from build123d import *

# Parameters (mm, degrees)
F1_DEPTH = 57.15
F2_R     = 3.175
F3_R     = 28.57499
F4_R     = 28.575
F5_R     = 28.57499
F7_D     = 15.875
F8_D     = 25.4
F8_DEPTH = 38.1
F8_TIP   = 7.6309298617
F9_D     = 25.4


# Not quite as in the source:
# - a fillet or chamfer is up to 0.001 mm smaller than in the source, because OpenCascade refuses the exact size
# - a length typed as a fraction of an inch, garbled in the dataset ("3 / 203.2 mm" for 3/8 in), is restored


with BuildPart() as f1:
    # F0 (on Top) → F1 (new body)
    with BuildSketch(Plane.XY):
        with BuildLine():
            ThreePointArc((28.575, -6.35), (30.4348719395, -1.8598719395), (34.925, 0))
            Line((34.925, 0), (609.6, 0))
            Line((609.6, 0), (609.6, 15.875))
            Line((609.6, 15.875), (34.925, 15.875))
            ThreePointArc((34.925, 15.875), (30.4348719395, 17.7348719395), (28.575, 22.225))
            Line((28.575, 22.225), (28.575, 36.5125))
            Line((28.575, 36.5125), (0, 36.5125))
            Line((0, 36.5125), (-28.575, 36.5125))
            Line((-28.575, 36.5125), (-28.575, 22.225))
            ThreePointArc((-28.575, 22.225), (-30.4348719395, 17.7348719395), (-34.925, 15.875))
            Line((-34.925, 15.875), (-304.8, 15.875))
            Line((-304.8, 15.875), (-304.8, 0))
            Line((-304.8, 0), (-34.925, 0))
            ThreePointArc((-34.925, 0), (-30.4348719395, -1.8598719395), (-28.575, -6.35))
            Line((-28.575, -6.35), (-28.575, -20.6375))
            Line((-28.575, -20.6375), (0, -20.6375))
            Line((0, -20.6375), (28.575, -20.6375))
            Line((28.575, -20.6375), (28.575, -6.35))
        make_face()
    extrude(amount=F1_DEPTH)

    # F2
    f2_edges = [f1.edges().sort_by_distance(p)[0] for p in [
        (28.575, 36.5125, 28.575),
        (0, 36.5125, 57.15),
        (-28.575, 36.5125, 28.575),
        (0, 36.5125, 0),
        (-28.575, -20.6375, 28.575),
        (0, -20.6375, 57.15),
        (28.575, -20.6375, 28.575),
        (0, -20.6375, 0),
    ]]
    fillet(f2_edges, radius=F2_R)

    # F3 (radius 28.575 in the source; OpenCascade refuses exactly that, so slightly less here)
    f3_edges = [f1.edges().sort_by_distance(p)[0] for p in [
        (-304.8, 7.9375, 57.15),
        (-304.8, 7.9375, 0),
    ]]
    fillet(f3_edges, radius=F3_R)

    # F4
    f4_edges = [f1.edges().sort_by_distance(p)[0] for p in [
        (609.6, 7.9375, 57.15),
    ]]
    fillet(f4_edges, radius=F4_R)

    # F5 (radius 28.575 in the source; OpenCascade refuses exactly that, so slightly less here)
    f5_edges = [f1.edges().sort_by_distance(p)[0] for p in [
        (609.6, 7.9375, 0),
    ]]
    fillet(f5_edges, radius=F5_R)

    # F7 (through all)
    with Locations(Plane.XZ):
        with Locations((-215.9, 28.575)):
            Hole(F7_D / 2)

    # F8 (one way)
    with BuildSketch(Plane.XZ):
        with Locations((0, 28.575)):
            Circle(F8_D / 2)
    extrude(amount=-F8_DEPTH, mode=Mode.SUBTRACT)
    with Locations(Plane.XZ):
        with Locations((0, 28.575)):
            with Locations((0, 0, -(F8_DEPTH + F8_TIP / 2))):  # 118° drill point
                Cone(0, F8_D / 2, F8_TIP, mode=Mode.SUBTRACT)

    # F9 (through all)
    with Locations(Plane(origin=(0, 0, 0), x_dir=(1, 0, 0), z_dir=(0, 1, 0))):
        with Locations((0, -28.575)):
            Hole(F9_D / 2)


solid = f1.part
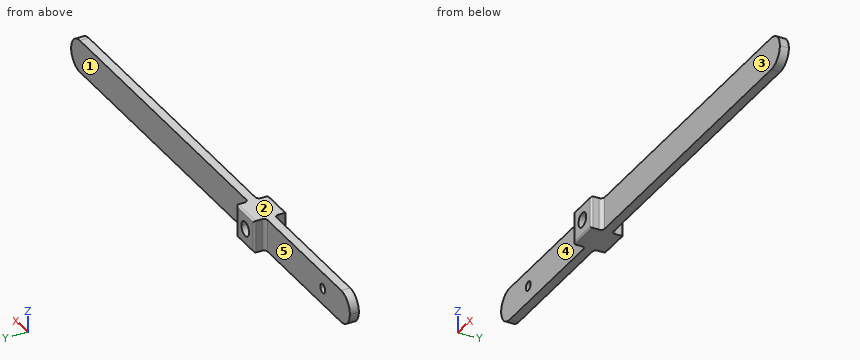
Source: CAD feature listing. Evaluate the final solid. Frame: model axes, mm. Face numbers are marked on the shaded views. A direction names the side the tool comes from. Round coordinates to 2 decimals unless told otherwise and drop trailing zeros. One line per item, written item: value. Start each with the question number.
Item 1: Ray query, L1, parallel to X at y = 7, z = 33.5; L2, parallel to Z at x = 0, y = -6 (3 decimals); L3, parallel to Z at x = -215.9, y = 9. Return the intervals inside material, ascending. Write a range as from..to.
Item 2: Pin query (flat end, axial travel): pin 1 (2 mm diameter, centred on x = 487.5, z = 29.5, fed in from -Y); pin 2 (6 mm diameter, centred on y = -9.5, z = 41, fed in from -X) (3 decimals); pin 3 (9.5 mm diameter, centred on x = -215.9, z = 28.575, fed in from -Y); pin 4 (5.5 mm diameter, centred on y = -9, z = 15.5, fed in from +X). Return the tip coordinate at first contact, or that it passes through.
Item 3: Set-up query: the marked faces 1, 2, 3, 4 and 5. Return all of +Z, -Z, +X, -X, +Y, -Y with unobstructed straight access to the full face (end or side cutting, diameter ignored); none if empty.
Result set:
1. L1: x = -304.37..-222.12, -209.68..-11.71, 11.71..609.17
1. L2: z = 0..15.875, 41.275..57.15
1. L3: z = 0..20.64, 36.51..57.15
2. pin 1: stops at y = 0
2. pin 2: stops at x = -28.575
2. pin 3: passes through
2. pin 4: stops at x = 28.58
3. face 1: +Z, -Z, +X, +Y
3. face 2: +Z, +X, -X, +Y, -Y
3. face 3: +Z, -Z, +X, -Y
3. face 4: +Z, -Z, -X, -Y
3. face 5: +Z, -Z, -X, +Y
